```python
from build123d import *

# Parameters (mm, degrees)
SKETCH1_R                    = 50
BOSS_EXTRUDE1_DEPTH          = 5
F_15_0_15_DIAMETER_HOLE1_D   = 15
F_10_2_10_2_DIAMETER_HOLE1_D = 10.2
M3_CLEARANCE_HOLE1_D         = 3.4
SKETCH9_R                    = 14.6
CUT_EXTRUDE1_DEPTH           = 10
SKETCH10_R                   = 4
CUT_EXTRUDE2_DEPTH           = 10


with BuildPart() as part:
    # Sketch1 → Boss-Extrude1 (new body)
    with BuildSketch(Plane.XY):
        Circle(SKETCH1_R)
    extrude(amount=BOSS_EXTRUDE1_DEPTH)

    # Ø15.0 (15) Diameter Hole1 (through all)
    with Locations(Plane(origin=(0, 0, 0), x_dir=(-1, 0, 0), z_dir=(0, 0, -1))):
        with Locations((0, 0)):
            Hole(F_15_0_15_DIAMETER_HOLE1_D / 2)

    # Ø10.2 (10.2) Diameter Hole1 (through all)
    with Locations(Plane(origin=(0, 0, 0), x_dir=(-1, 0, 0), z_dir=(0, 0, -1))):
        with Locations((37, 0), (-37, 0), (0, -40)):
            Hole(F_10_2_10_2_DIAMETER_HOLE1_D / 2)

    # M3 Clearance Hole1 (through all)
    with Locations(Plane.XY.offset(5)):
        with Locations((46, 0), (28, 0), (9, -40), (-9, -40), (-46, 0), (-28, 0)):
            Hole(M3_CLEARANCE_HOLE1_D / 2)

    # Sketch9 → Cut-Extrude1 (cut)
    with BuildSketch(Plane.XY.offset(5)):
        with Locations((24.04163056, -24.04163056)):
            Circle(SKETCH9_R)
        with Locations((-24.04163056, -24.04163056)):
            Circle(SKETCH9_R)
        with Locations((0, 34)):
            Circle(SKETCH9_R)
    extrude(amount=-CUT_EXTRUDE1_DEPTH, mode=Mode.SUBTRACT)

    # Sketch10 → Cut-Extrude2 (cut)
    with BuildSketch(Plane.XY.offset(5)):
        with Locations((28.284271247, 28.284271247)):
            Circle(SKETCH10_R)
    extrude(amount=-CUT_EXTRUDE2_DEPTH, mode=Mode.SUBTRACT)


solid = part.part
```
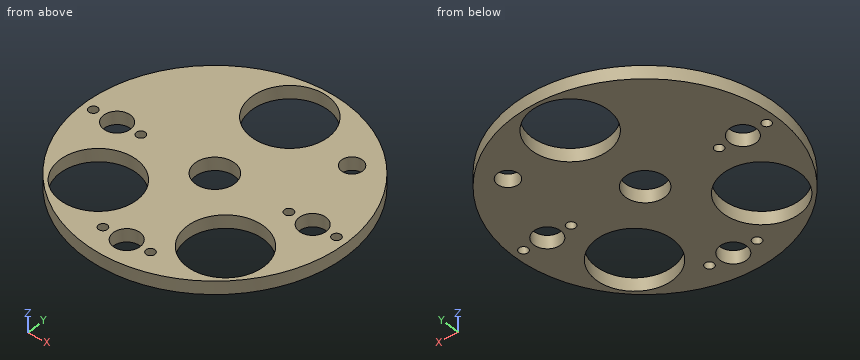
Model file for the job. Use its own axes, mm. Round coordinates to 2 decimals unless told otherwise and drop trailing zeros. Order: outer loops, then holes, each group sorted by start corner. A loop starts at its lowest first (then second) coordinate and runs counter-clockwise, first axis right, second up. Notation, with made-up numbers: M 8,41 L 57,41 A15 ccw 57,68 Z; hole C -33,-37.75 d7. An arc over 180 degrees is marked long. Use CSV: the item, a comma, the result in double quotes.
Item 1: Saw through at A-A (y = 0). State how many separate pieces and enclosed holes the cut face has, plus the area to 3 significant figures.
Worked answers:
separate pieces,"8"
enclosed holes,"0"
area,"255 mm²"
Item 2: Probe probe 1 along Y at (x, z) = (31.5, 0.9); probe 2 along X at (y, z) = (-28, 0.7); probe 3 along Y at (x, z) = (35.5, 0.55). List the from-to ranges inside material, lowest first.
Worked answers:
probe 1,"-38.83 to -36.59, -11.49 to 25.91, 30.66 to 38.83"
probe 2,"-41.42 to -38.09, -9.99 to 9.99, 38.09 to 41.42"
probe 3,"-35.21 to -33.09, -14.99 to -4.87, 4.87 to 35.21"
Item 3: Saw through at D-D (x = -28). List the corners of the cut face in (y, z).
Worked answers:
outline,"M -41.42,0 L -38.09,0 L -38.09,5 L -41.42,5 Z; M -9.99,0 L -1.7,0 L -1.7,5 L -9.99,5 Z; M 1.7,0 L 41.42,0 L 41.42,5 L 1.7,5 Z"
Item 4: Saw through at B-B (y = -40). List the corners of the cut face in (x, z), plus the area to 3 significant figures.
Worked answers:
outline,"M -30,0 L -10.7,0 L -10.7,5 L -30,5 Z; M -7.3,0 L -5.1,0 L -5.1,5 L -7.3,5 Z; M 5.1,0 L 7.3,0 L 7.3,5 L 5.1,5 Z; M 10.7,0 L 30,0 L 30,5 L 10.7,5 Z"
area,"215 mm²"
Item 5: Saw through at C-C (x = -46). List the corners of the cut face in (y, z), plus the area to 3 significant figures.
Worked answers:
outline,"M -19.6,0 L -1.7,0 L -1.7,5 L -19.6,5 Z; M 1.7,0 L 19.6,0 L 19.6,5 L 1.7,5 Z"
area,"179 mm²"
Item 6: Pin check, flat tips, straight feed: pin 1 (2 mm diameter, centred on x = -46, y = 0, fed in from +Z); pin 2 (2 mm diameter, centred on y = 21.5, z = 4.5, fed in from +X); pin 3 (2 mm diameter, centred on y = -21, z = 3, fed in from -X). Stop position of each tip, or through.
Worked answers:
pin 1,"through"
pin 2,"x = 45.6"
pin 3,"x = -45.83"
